Check sheet for the drawn part. Datum: minimum x, y, z corner. Units: mm. Coordinates: 2 decimals unless noted, no trailing zeros. Order: outer loops, then holes, each group sorted by start corner. A loop starts at its lowest first (then second) coordinate and runs counter-clockwise, first axis right, second up. Notation, with made-up numbers: M -29.75,49.5 L -4.75,49.5 A10 ccw -4.75,68.5 Z; hole C 6.5,87.5 d11. An arc over 180 degrees is marked long. Return JSON: item names as keys, results as strings. Group by question number.
Q1. Section check A-A, the plane z = 31. Enter the section's corners in (x, y).
Q2. Section check C-C, the plane z = 19. Enter the section's corners in (x, y), then the cut area to 3 significant figures.
Q3. Section check D-D, the plane y = 0.55. Enter the section's corners in (x, z), then the cut area to 3 significant figures.
Q4. Thickness scan on probe 1 along X at (y, z) = (0.3, 7.5); probe 2 along Z at (x, y) = (104, 1.6); probe 3 along X at (y, z) = (0.65, 17) (1 decimal). Record the ranges inside material, lowest first.
Q5. Section check B-B, the plane x = 104. Enter the section's corners in (y, z).
Q6. Go/stop test with flat-tipped pins: pin 1 Ø1.5 at (x, y) = (68, 1) entering from -Z; pin 2 Ø1.5 at (y, z) = (1, 1.5) entering from +X; pin 3 Ø0.9 at (y, z) = (1.5, 38.5) entering from +X. Record where each tip stops, or that it passes through.
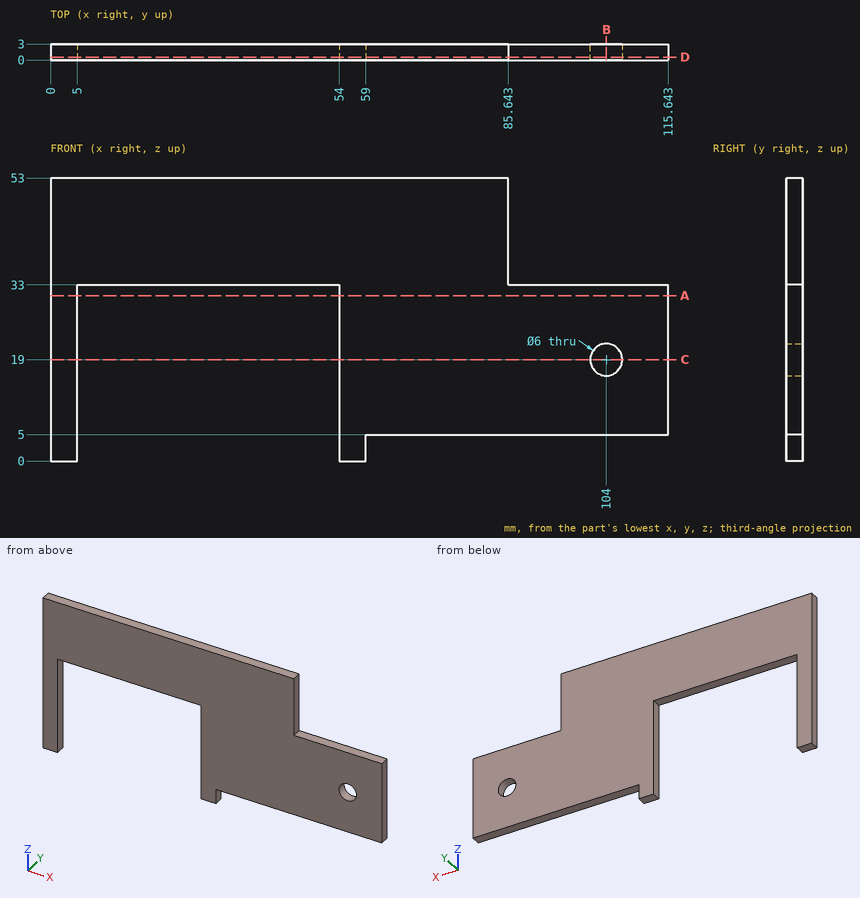
Numbers:
{
 "1": {"outline": "M 0,0 L 5,0 L 5,3 L 0,3 Z; M 54,0 L 115.64,0 L 115.64,3 L 54,3 Z"},
 "2": {"outline": "M 0,0 L 5,0 L 5,3 L 0,3 Z; M 54,0 L 101,0 L 101,3 L 54,3 Z; M 107,0 L 115.64,0 L 115.64,3 L 107,3 Z", "area": "182 mm2"},
 "3": {"outline": "M 0,0 L 5,0 L 5,33 L 54,33 L 54,0 L 59,0 L 59,5 L 115.64,5 L 115.64,33 L 85.64,33 L 85.64,53 L 0,53 Z; hole C 104,19 d6", "area": "3,600 mm2"},
 "4": {"probe 1": "x = 0 to 5, 54 to 115.64", "probe 2": "z = 5 to 16, 22 to 33", "probe 3": "x = 0 to 5, 54 to 101.8, 106.2 to 115.6"},
 "5": {"outline": "M 0,5 L 3,5 L 3,16 L 0,16 Z; M 0,22 L 3,22 L 3,33 L 0,33 Z"},
 "6": {"pin 1": "stops at z = 5", "pin 2": "stops at x = 59", "pin 3": "stops at x = 85.64"}
}
